```python
from build123d import *

# Parameters (mm, degrees)
SKETCH_1_W          = 7
SKETCH_1_H          = 4.5
EXTRUDE_1_DEPTH     = 3.5
SKETCH_3_W          = 3
SKETCH_3_H          = 3
EXTRUDE_2_DEPTH     = 6.5
SKETCH_4_W          = 1.6
SKETCH_4_H          = 0.5
CUT_EXTRUDE_1_DEPTH = 10.813893213
CUT_EXTRUDE_2_DEPTH = 6.5
FILLET_1_R          = 0.1


with BuildPart() as part:
    # 草图1 → 凸台-拉伸1 (new body)
    with BuildSketch(Plane.XY):
        Rectangle(SKETCH_1_W, SKETCH_1_H)
    extrude(amount=EXTRUDE_1_DEPTH)

    # 草图3 → 凸台-拉伸2 (add)
    with BuildSketch(Plane(origin=(0, 0, 0), x_dir=(-1, 0, 0), z_dir=(0, 0, -1))):
        Rectangle(SKETCH_3_W, SKETCH_3_H)
    extrude(amount=EXTRUDE_2_DEPTH)

    # 草图4 → 切除-拉伸1 (cut, through all)
    with BuildSketch(Plane(origin=(3.5, 0, 0), x_dir=(0, 0, -1), z_dir=(1, 0, 0))):
        with Locations((-3.5, 0)):
            Rectangle(SKETCH_4_W, SKETCH_4_H)
    extrude(amount=-CUT_EXTRUDE_1_DEPTH, mode=Mode.SUBTRACT)

    # 草图5 → 切除-拉伸2 (cut)
    with BuildSketch(Plane(origin=(0, 1.5, 0), x_dir=(1, 0, 0), z_dir=(0, 1, 0))):
        Polygon((-0.65, 6.5), (-1.3, 6.5), (-0.975, 6.2), align=None)
        Polygon((0, 6.5), (-0.65, 6.5), (-0.325, 6.2), align=None)
        Polygon((0.65, 6.5), (0, 6.5), (0.325, 6.2), align=None)
        Polygon((1.3, 6.5), (0.65, 6.5), (0.975, 6.2), align=None)
    extrude(amount=-CUT_EXTRUDE_2_DEPTH, mode=Mode.SUBTRACT)

    # 圆角1
    fillet_1_edges = [part.edges().sort_by_distance(p)[0] for p in [
        (1.5, 0, -6.5),
        (-1.5, 0, -6.5),
        (0.65, 0, -6.5),
        (0, 0, -6.5),
        (-0.65, 0, -6.5),
        (-1.3, 0, -6.5),
        (-0.975, 0, -6.2),
        (0.325, 0, -6.2),
        (-0.325, 0, -6.2),
        (1.3, 0, -6.5),
        (0.975, 0, -6.2),
    ]]
    fillet(fillet_1_edges, radius=FILLET_1_R)


solid = part.part
```
Geometry: final body of the model. Coordinates: model frame, mm. A direction names the side the tool comes from. Round coordinates to 2 decimals unless told otherwise and drop trailing zeros. Loops run counter-clockwise (first coordinate to the right, second up) from the corner with the lowest first, then second, coordinate; pieces in that order, holes last. Notation, with made-up numbers: (-3, 56) -> (24, 56) arc R27 cw to (24, 89) -> close; hole circle Ø4 at (87.25, 17.5). An arc over 180 degrees is marked (long way). Use one line per item in the form item = value.
Item 1: Cut plane A-A on y = 0.7. Output: boundary loops of the cut face in (x, z) (3 decimals).
Evaluation:
outline = (-3.5, 0) -> (-1.5, 0) -> (-1.5, -6.4) arc R0.1 ccw to (-1.4, -6.5) -> (-1.339, -6.5) arc R0.1 ccw to (-1.271, -6.473) -> (-1.043, -6.263) arc R0.1 cw to (-0.907, -6.263) -> (-0.718, -6.437) arc R0.1 ccw to (-0.582, -6.437) -> (-0.393, -6.263) arc R0.1 cw to (-0.257, -6.263) -> (-0.068, -6.437) arc R0.1 ccw to (0.068, -6.437) -> (0.257, -6.263) arc R0.1 cw to (0.393, -6.263) -> (0.582, -6.437) arc R0.1 ccw to (0.718, -6.437) -> (0.907, -6.263) arc R0.1 cw to (1.043, -6.263) -> (1.271, -6.473) arc R0.1 ccw to (1.339, -6.5) -> (1.4, -6.5) arc R0.1 ccw to (1.5, -6.4) -> (1.5, 0) -> (3.5, 0) -> (3.5, 3.5) -> (-3.5, 3.5) -> close
Item 2: Access query for faces 1 (the flat face through (-1.5, 0, -3)), 2 (the flat face through (0, -1.5, -3)), 3 (the flat face through (0, -1, 3.5)), 4 (the flat face through (0, 1.5, -3)), 5 (the flat face through (1.5, 0, -3)). Directions: +Z, -Z, +X, -X, +Y, -Y. A direction counts if a zero-diameter tool reaches every point of the face in a straight line with its end or side. Return the directions, or none.
Evaluation:
face_1 = -Z, -X, +Y, -Y
face_2 = -Z, +X, -X, -Y
face_3 = +Z, +X, -X, +Y, -Y
face_4 = -Z, +X, -X, +Y
face_5 = -Z, +X, +Y, -Y
Item 3: Material intervals for probe 1 along Y at (x, z) = (-1.25, -4); probe 2 along Z at (x, y) = (1, 0); probe 3 along Z at (x, y) = (2.75, 1.65), sorted ascending.
Evaluation:
probe_1 = -1.5 to 1.5
probe_2 = -6.24 to 2.7
probe_3 = 0 to 3.5
Item 4: Cut plane C-C on z = -2.5. Output: boundary loops of the cut face in (x, y), then the cut area to 3 significant figures.
Evaluation:
outline = (-1.5, -1.5) -> (1.5, -1.5) -> (1.5, 1.5) -> (-1.5, 1.5) -> close
area = 9.00 mm2
Item 5: Cut plane B-B on x = 2. Output: boundary loops of the cut face in (y, z), then the cut area to 4 significant figures.
Evaluation:
outline = (-2.25, 0) -> (2.25, 0) -> (2.25, 3.5) -> (0.25, 3.5) -> (0.25, 2.7) -> (-0.25, 2.7) -> (-0.25, 3.5) -> (-2.25, 3.5) -> close
area = 15.35 mm2
Item 6: Contact query for flat-ended pins moving along their axis: pin 1 Ø1.5 at (x, z) = (-0.5, -3.5) entering from +Y; pin 2 Ø2.5 at (x, z) = (0, -2) entering from -Y. Output: stop coordinate, or through.
Evaluation:
pin_1 = 1.5
pin_2 = -1.5
